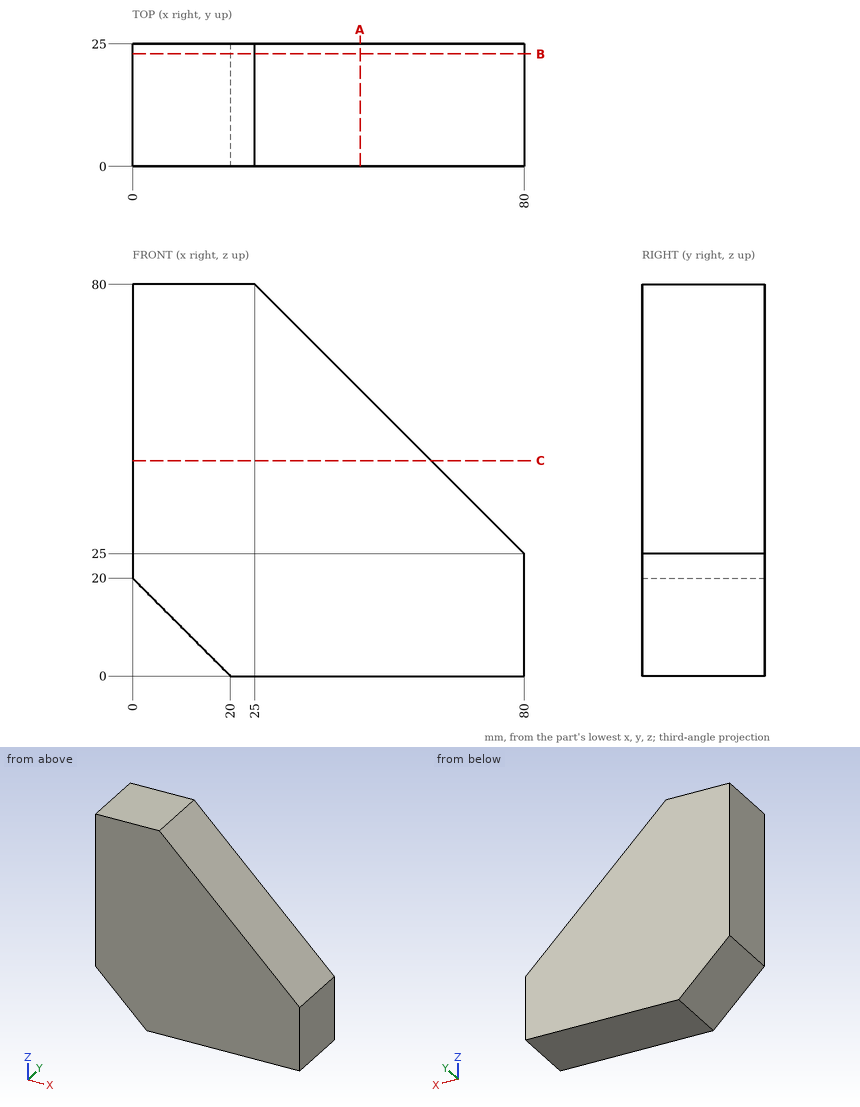
Input: dimensioned drawing with shaded views. Units: mm. Origin: part minimum x, y, z. Give positions to 0.01 mm unless a question says otherwise; leave off trailing zeros. Write each loop counter-clockwise with the first axis right and the second up, starting at its lowest first coordinate (ties: lowest second). Pieces come first, ordered by that corner, then holes.
Q1. Section B-B, the plane y = 23. Output: boundary loops of the cut face in (x, z), plus the area to 3 significant figures.
Q2. Material intervals for probe 1 along Z at (x, y) = (69.5, 18.5); probe 2 along X at (y, z) = (16.5, 36.5); probe 3 along X at (y, z) = (11.75, 4), sorted ascending.
Q3. Section A-A, the plane x = 46.5. Output: boundary loops of the cut face in (y, z), plus the area to 3 significant figures.
Q4. Section C-C, the plane z = 44. Output: boundary loops of the cut face in (x, y).
Q5. First-contact query: P1, Ø10, axis at x = 31, z = 30, coming from the -Y side; P2, Ø6, axis at x = 62, y = 20.5, coming from the +Z side; P3, Ø2, axis at y = 4, z = 40.5, coming from the +X side; P4, Ø3, axis at y = 12, z = 34.5, coming from the +X side. Flat tips, straight axial feed; report the tip coordinate or a pass-through.
Filled in:
1. outline: (0, 20) - (20, 0) - (80, 0) - (80, 25) - (25, 80) - (0, 80) - close
1. area: 4,690 mm2
2. probe 1: z = 0 to 35.5
2. probe 2: x = 0 to 68.5
2. probe 3: x = 16 to 80
3. outline: (0, 0) - (25, 0) - (25, 58.5) - (0, 58.5) - close
3. area: 1,460 mm2
4. outline: (0, 0) - (61, 0) - (61, 25) - (0, 25) - close
5. P1: stops at y = 0
5. P2: stops at z = 46
5. P3: stops at x = 65.5
5. P4: stops at x = 72
